Input: dimensioned drawing with shaded views. Units: mm. Origin: part minimum x, y, z. Give positions to 0.01 mm unless a question says otherwise; leave off trailing zeros. Write each loop counter-clockwise with the first axis right and the second up, starting at its lowest first coordinate (ties: lowest second). Pieces come first, ordered by that corner, then holes.
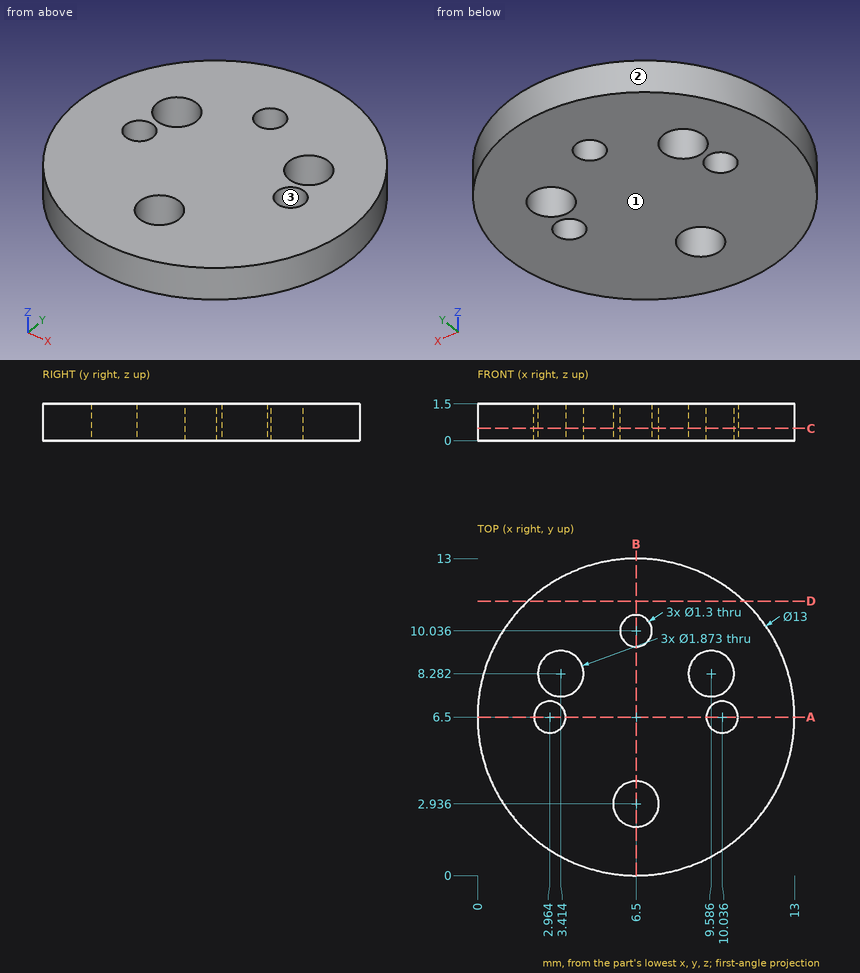
1. Cut plane C-C, the plane z = 0.5. State how many separate pieces and enclosed holes the cut face has.
2. Cut plane B-B, the plane x = 6.5. Return the cut outline in (y, z) (1 decimal).
3. Cut plane A-A, the plane y = 6.5. Return the cut outline in (x, z) (1 decimal), then the cut area to 3 significant figures.
4. Mould query, pull axis Y, two halves, no side actions, for the marked faces 1, 2 and 3. Classes: +Y half, -Y half, draft (parallel to the pull), parting line (faces both ways), or undercut.
5. Line query: L1, parallel to Y at x = 6.5, z = 0.55 (1 decimal); L2, parallel to Y at x = 6.25, z = 1.45 (1 decimal); L3, parallel to X at y = 8.5, z = 1 (1 decimal). Output: solid intervals per line, ascending.
6. Cut plane D-D, the plane y = 11.25. Return the cut outline in (x, z), then the cut area to 3 significant figures.
Response values:
1. separate pieces: 1
1. enclosed holes: 6
2. outline: (0, 0) - (2, 0) - (2, 1.5) - (0, 1.5) - close; (3.9, 0) - (9.4, 0) - (9.4, 1.5) - (3.9, 1.5) - close; (10.7, 0) - (13, 0) - (13, 1.5) - (10.7, 1.5) - close
3. outline: (0, 0) - (2.3, 0) - (2.3, 1.5) - (0, 1.5) - close; (3.6, 0) - (9.4, 0) - (9.4, 1.5) - (3.6, 1.5) - close; (10.7, 0) - (13, 0) - (13, 1.5) - (10.7, 1.5) - close
3. area: 15.6 mm2
4. face 1: draft
4. face 2: parting line
4. face 3: undercut
5. L1: y = 0 to 2, 3.9 to 9.4, 10.7 to 13
5. L2: y = 0 to 2, 3.8 to 9.4, 10.6 to 13
5. L3: x = 0.3 to 2.5, 4.3 to 8.7, 10.5 to 12.7
6. outline: (2.06, 0) - (10.94, 0) - (10.94, 1.5) - (2.06, 1.5) - close
6. area: 13.3 mm2
